Source: CAD feature listing. Evaluate the final solid. Frame: model axes, mm. Face numbers are marked on the shaded views. A direction names the side the tool comes from. Coordinates: 2 decimals unless noted, no trailing zeros. Loops run counter-clockwise (first coordinate to the right, second up) from the corner with the lowest first, then second, coordinate; pieces in that order, holes last. Notation, with made-up numbers: (-31, 41) - (20, 41) arc R15 ccw to (20, 65) - close; hole circle Ø9 at (-31, -13). An arc over 180 degrees is marked (long way). Write item = value, one per line. Start each with the question number.
from build123d import *

# Parameters (mm, degrees)
SKETCH1_R           = 2
BOSS_EXTRUDE1_DEPTH = 5
SKETCH1_4_R         = 5.85
SKETCH1_4_R_2       = 4.85
EXTRUDE_THIN1_DEPTH = 20


with BuildPart() as part:
    # Sketch1 → Boss-Extrude1 (new body)
    with BuildSketch(Plane.XY):
        with BuildLine():
            Line((2.96969697, 19.045454545), (42.96969697, 19.045454545))
            ThreePointArc((42.96969697, 19.045454545), (46.505230876, 17.580988451), (47.96969697, 14.045454545))
            Line((47.96969697, 14.045454545), (47.96969697, 4.045454545))
            ThreePointArc((47.96969697, 4.045454545), (46.505230876, 0.50992064), (42.96969697, -0.954545455))
            Line((42.96969697, -0.954545455), (3.116761061, -0.954545455))
            ThreePointArc((3.116761061, -0.954545455), (-0.522762861, 0.552994715), (-2.03030303, 4.192518637))
            Line((-2.03030303, 4.192518637), (-2.03030303, 14.045454545))
            ThreePointArc((-2.03030303, 14.045454545), (-0.565836936, 17.580988451), (2.96969697, 19.045454545))
        make_face()
        with Locations((22.96969697, 9.082220568)):
            Circle(SKETCH1_R, mode=Mode.SUBTRACT)
    extrude(amount=BOSS_EXTRUDE1_DEPTH)

    # Sketch1<4> → Extrude-Thin1 (add)
    with BuildSketch(Plane.XY):
        with Locations((7.969686156, 9.104280198)):
            Circle(SKETCH1_4_R)
        with Locations((7.969686156, 9.104280198)):
            Circle(SKETCH1_4_R_2, mode=Mode.SUBTRACT)
        with Locations((37.96969697, 9.060160955)):
            Circle(SKETCH1_4_R)
        with Locations((37.96969697, 9.060160955)):
            Circle(SKETCH1_4_R_2, mode=Mode.SUBTRACT)
    extrude(amount=EXTRUDE_THIN1_DEPTH)


solid = part.part
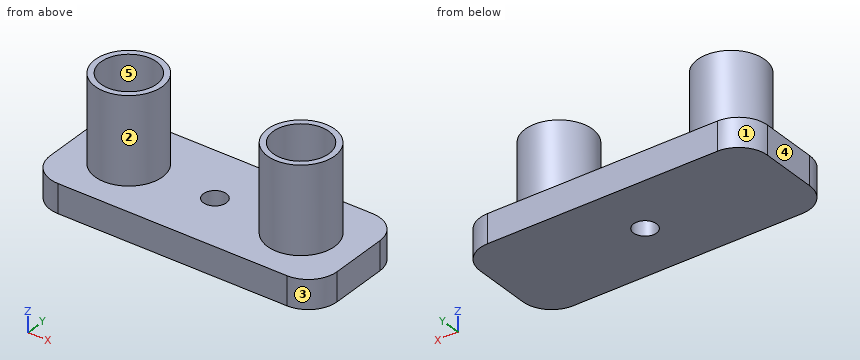
Item 1: Material intervals for L1, parallel to Y at x = 8, z = 9; L2, parallel to X at y = 11.75, z = 11.5; L3, parallel to X at y = 6.25, z = 11.25, sorted ascending. Write a range as [from, to].
Item 2: Cut plane C-C (z = 1). Return the cut outline in (x, y), then the cut area to 3 significant figures.
Item 3: Cut plane B-B (y = 4.75). Return the cut outline in (x, z), then the cut area to 3 significant figures.
Item 4: Cut plane A-A (z = 6.5). Return the cut outline in (x, y), then the cut area to 3 significant figures.
Item 5: Cut plane D-D (x = 7.5). Return the cut outline in (y, z), then the cut area to 3 significant figures.
Item 6: Reachability of the marked faces 1 and 2 from +Z, -Z, +X, -X, +Y, -Y: full face, straight path, thin tool, end or side. Return the list, or none.
Item 7: Draft query along Y for the marked faces 3, 4 and 5. Return one class per face: released by +Y, released by -Y, zero draft, split by the parting line, or undercut.
Item 8: First-contact query: pin 1 (4.5 mm diameter, centred on x = 22.97, y = 9.08, fed in from +Z); pin 2 (8 mm diameter, centred on x = 16, y = 5.5, fed in from +Z); pin 3 (1 mm diameter, centred on x = 41.5, z = 9.5, fed in from -Y); pin 4 (10 mm diameter, centred on x = 23, z = 15.5, fed in from -Y). Flat tips, straight axial feed; report the tip coordinate or a pass-through.
Responses:
q1.L1 = [3.25, 4.25], [13.95, 14.95]
q1.L2 = [2.75, 3.9], [12.03, 13.19], [32.77, 33.93], [42.01, 43.16]
q1.L3 = [2.86, 4.05], [11.89, 13.08], [32.84, 34.02], [41.92, 43.1]
q2.outline = (-2.03, 4.19) arc R5.15 ccw to (3.12, -0.95) - (42.97, -0.95) arc R5 ccw to (47.97, 4.05) - (47.97, 14.05) arc R5 ccw to (42.97, 19.05) - (2.97, 19.05) arc R5 ccw to (-2.03, 14.05) - close; hole circle Ø4 at (22.97, 9.08)
q2.area = 966 mm2
q3.outline = (-2.03, 0) - (47.97, 0) - (47.97, 5) - (41.93, 5) - (41.93, 20) - (40.19, 20) - (40.19, 5) - (35.75, 5) - (35.75, 20) - (34.01, 20) - (34.01, 5) - (11.88, 5) - (11.88, 20) - (10.11, 20) - (10.11, 5) - (5.83, 5) - (5.83, 20) - (4.06, 20) - (4.06, 5) - (-2.03, 5) - close
q3.area = 355 mm2
q4.outline = circle Ø11.7 at (7.97, 9.1); circle Ø11.7 at (37.97, 9.06); hole circle Ø9.7 at (7.97, 9.1); hole circle Ø9.7 at (37.97, 9.06)
q4.area = 67.2 mm2
q5.outline = (-0.95, 0) - (19.05, 0) - (19.05, 5) - (14.94, 5) - (14.94, 20) - (13.93, 20) - (13.93, 5) - (4.28, 5) - (4.28, 20) - (3.27, 20) - (3.27, 5) - (-0.95, 5) - close
q5.area = 130 mm2
q6.face_1 = +Z, -Z, -X, +Y
q6.face_2 = +Z
q7.face_3 = released by -Y
q7.face_4 = zero draft
q7.face_5 = undercut
q8.pin_1 = 5
q8.pin_2 = 20
q8.pin_3 = 4.06
q8.pin_4 = through
